Autodesk Inventor part; units mm, degrees
ref_plane "YZ Plane" through (0, 0, 0) normal (1, 0, 0) x (0, 1, 0)
ref_plane "XZ Plane" through (0, 0, 0) normal (0, 1, 0) x (-1, 0, 0)
ref_plane "XY Plane" through (0, 0, 0) normal (0, 0, 1) x (1, 0, 0)
sketch "Esquisse1" plane through (0, 0, 0) normal (0, 1, 0) x (-1, 0, 0)
  line L0 (-90, 100) -> (90, 100)
  line L1 (90, 100) -> (90, -100)
  line L2 (90, -100) -> (-90, -100)
  line L3 (-90, -100) -> (-90, 100)
  line L4 (-90, 100) -> (90, -100) construction
  line L5 (90, 100) -> (-90, -100) construction
  point P0 (0, 0)
  dimension "d0" = 180
  dimension "d1" = 200
extrude "Extrusion1" add sketch "Esquisse1" along normal blind 5
sketch "Esquisse2" plane through (0, 5, 0) normal (0, 1, 0) x (1, 0, 0)
  line L0 (0, 0) -> (0, -97.5)
  line L1 (0, -97.5) -> (-87.5, -97.5)
  line L2 (0, 0) -> (-32.0024, 0)
  point P0 (87.5, -97.5)
  point P1 (-87.5, 97.5)
  point P2 (87.5, 97.5)
  dimension "d4" = 97.5
  dimension "d5" = 87.5
hole "Perçage1" at (-87.5, 5, 97.5) at (87.5, 5, 97.5) at (-87.5, 5, -97.5) at (87.5, 5, -97.5) direction (0, -1, 0) diameter 2.459 end through all
sketch "Esquisse3" plane through (0, 5, 0) normal (0, 1, 0) x (1, 0, 0)
  line L0 (0, 0) -> (-87.5, 0)
  line L1 (0, 0) -> (0, 97.5)
  point P0 (87.5, 0)
  point P1 (0, -97.5)
  dimension "d13" = 87.5
  dimension "d14" = 97.5
hole "Perçage2" at (-87.5, 5, 0) at (0, 5, -97.5) at (87.5, 5, 0) at (0, 5, 97.5) direction (0, -1, 0) diameter 2.459 end through all
sketch "Esquisse4" plane through (0, 5, 0) normal (0, 1, 0) x (1, 0, 0)
  line L0 (0, 0) -> (0, 40)
  dimension "d22" = 40
hole "Perçage3" at (0, 5, -40) direction (0, -1, 0) diameter 5.9175 end through all
properties part number "chassis_haut"
For this review, take the finished solid that the model builds, in its own axes (mm). Round coordinates to 2 decimals unless told otherwise and drop trailing zeros. Loops run counter-clockwise (first coordinate to the right, second up) from the corner with the lowest first, then second, coordinate; pieces in that order, holes last. Notation, with made-up numbers: (55, 19) - (105, 19) arc R32 cw to (105, 50) - close; hole circle Ø2 at (29.5, 35). An arc over 180 degrees is marked (long way). One line per item, written item: value. Start each with the question number.
Item 1: The part is to be moulded in two halves that separate along X. For faces 1 (the flat face through (90, 2, -1)), 2 (the flat face through (-1, 2, -100)), 3 (the cylindrical face through (-0.13, 2.465, -42.956)), say which applies: +X half, -X half, draft (parallel to the pull), parting line (faces both ways), or undercut.
Item 2: For L1, parallel to Z at x = 0, y = 3.55; L2, parallel to X at y = 2.35, z = 0; L3, parallel to X at y = 3.85, z = -97.5, list the stretches that pass through material, from the lowest coordinate up.
Item 3: Take a section at A-A (z = -40). Give the boundary of the cut face in (x, y).
Answer below:
1. face 1: +X half
1. face 2: draft
1. face 3: undercut
2. L1: z = -100 to -98.73, -96.27 to -42.96, -37.04 to 96.27, 98.73 to 100
2. L2: x = -90 to -88.73, -86.27 to 86.27, 88.73 to 90
2. L3: x = -90 to -88.73, -86.27 to -1.23, 1.23 to 86.27, 88.73 to 90
3. outline: (-90, 0) - (-2.96, 0) - (-2.96, 5) - (-90, 5) - close; (2.96, 0) - (90, 0) - (90, 5) - (2.96, 5) - close
